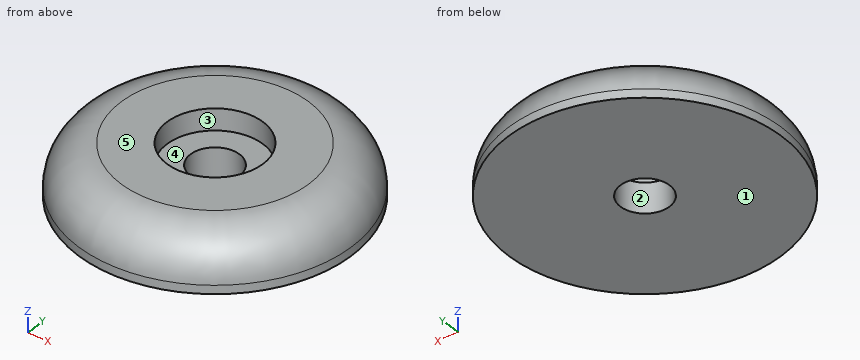
from build123d import *

# Parameters (mm, degrees)
F0_R     = 6.4
F0_R_2   = 1.15
F1_DEPTH = 2.4
F2_R     = 2.25
F3_DEPTH = 1
F4_R     = 2


with BuildPart() as f1:
    # F0 (on Top) → F1 (new body)
    with BuildSketch(Plane.XY):
        Circle(F0_R)
        Circle(F0_R_2, mode=Mode.SUBTRACT)
    extrude(amount=F1_DEPTH)

    # F2 (on face) → F3 (cut)
    with BuildSketch(Plane.XY.offset(2.4)):
        Circle(F2_R)
    extrude(amount=-F3_DEPTH, mode=Mode.SUBTRACT)

    # F4
    f4_edges = [f1.edges().sort_by_distance(p)[0] for p in [
        (-6.4, 0, 2.4),
    ]]
    fillet(f4_edges, radius=F4_R)


solid = f1.part
For this review, take the finished solid that the model builds, in its own axes (mm). Face numbers are marked on the shaded views. A direction names the side the tool comes from. Round coordinates to 2 decimals unless told otherwise and drop trailing zeros. Write each loop counter-clockwise with the first axis right and the second up, starting at its lowest first coordinate (ties: lowest second). Pieces come first, ordered by that corner, then holes. Notation, with made-up numbers: M -14,46 L 38,46 A24 cw 38,63 Z; hole C 29,-6.5 d10. An arc over 180 degrees is marked long. Write item = value, one per line. Start each with the question number.
(1) We need section C-C (z = 1.6). Give the boundary of the cut face in (x, y).
(2) We need section D-D (z = 0.9). Give the boundary of the cut face in (x, y).
(3) For line 1 along Y through (x, z) = (0, 0.4); line 2 along X through (y, z) = (-1, 0.6); line 3 along X through (y, z) = (1.25, 2.15), list the stretches that pass through material, from the lowest coordinate up.
(4) Clearance check with flat-ended pins moving along their axes: pin 1 Ø2 at (x, y) = (-0.5, -0.5) entering from +Z; pin 2 Ø1 at (y, z) = (5, 2) entering from -X. State where each tip first meets the part, or that it passes through.
(5) We need section A-A (x = 0). Give the boundary of the cut face in (y, z), then the cut area to 3 significant figures.
(6) The part is to be moulded in two halves that separate along X. For the marked faces 1, 2 and 3, say which applies: +X half, -X half, draft (parallel to the pull), parting line (faces both ways), or undercut.
(7) For the marked faces 4 and 5, list the 3-axis set-ups (+Z, -Z, +X, -X, +Y, -Y) from which the entire face can be reached by the end or side of a thin tool; tool diameter is ignored.
Results found:
q1.outline = C 0,0 d12; hole C 0,0 d4.5
q2.outline = C 0,0 d12.67; hole C 0,0 d2.3
q3.line_1 = -6.4 to -1.15, 1.15 to 6.4
q3.line_2 = -6.31 to -0.57, 0.57 to 6.31
q3.line_3 = -5.22 to -1.87, 1.87 to 5.22
q4.pin_1 = 1.4
q4.pin_2 = -3.74
q5.outline = M -6.4,0 L -1.15,0 L -1.15,1.4 L -2.25,1.4 L -2.25,2.4 L -4.4,2.4 A2 ccw -6.4,0.4 Z; M 1.15,0 L 6.4,0 L 6.4,0.4 A2 ccw 4.4,2.4 L 2.25,2.4 L 2.25,1.4 L 1.15,1.4 Z
q5.area = 21.3 mm²
q6.face_1 = draft
q6.face_2 = undercut
q6.face_3 = undercut
q7.face_4 = +Z
q7.face_5 = +Z, +X, -X, +Y, -Y
